Part print with two shaded views. Sizes in mm from the minimum x, y, z corner. A direction names the side the tool comes from. Give positions to 0.01 mm unless a question says otherwise; leave off trailing zeros. Write each loop counter-clockwise with the first axis right and the second up, starting at its lowest first coordinate (ties: lowest second). Pieces come first, ordered by that corner, then holes. Notation, with made-up numbers: M 64,80.25 L 73,80.25 A24 ccw 73,100.25 Z; hole C -39.5,42 d11. An arc over 180 degrees is marked long. Return JSON: item names as keys, results as strings. Group by question number.
Q1. Wall check: probe 1 along X at (y, z) = (1, 3); probe 2 along X at (y, z) = (3.75, 3); probe 3 along Z at (x, y) = (14, 3.5). Give the ranges that are in metal, low to high.
Q2. Band-saw the part on D-D, the plane x = 3.5. Give the cut face in (y, z), then the cut area to 3 significant figures.
Q3. Tool access for the marked faces 4, 5 and 6: list every direction of +Z, -Z, +X, -X, +Y, -Y with a clear straight run to the whole face (end or side of a thin tool).
Q4. Band-saw the part on C-C, the plane z = 3.25. Give the cut face in (x, y).
Q5. Pull direction Z, two halves, no side cores. Call the marked faces 1, 2 and 3: +Z half, -Z half, draft (parallel to the pull), parting line (faces both ways), or undercut.
Q6. Flat gauge pins, fed straight in: pin 1 Ø1.5 at (x, y) = (5.5, 6) entering from -Z; pin 2 Ø5 at (x, y) = (6, 5) entering from +Z; pin 3 Ø1 at (x, y) = (6, 4.5) entering from -Z. Where does each tip first touch, or does it go through?
Q7. Band-saw the part on B-B, the plane y = 4.25. Give the cut face in (x, z).
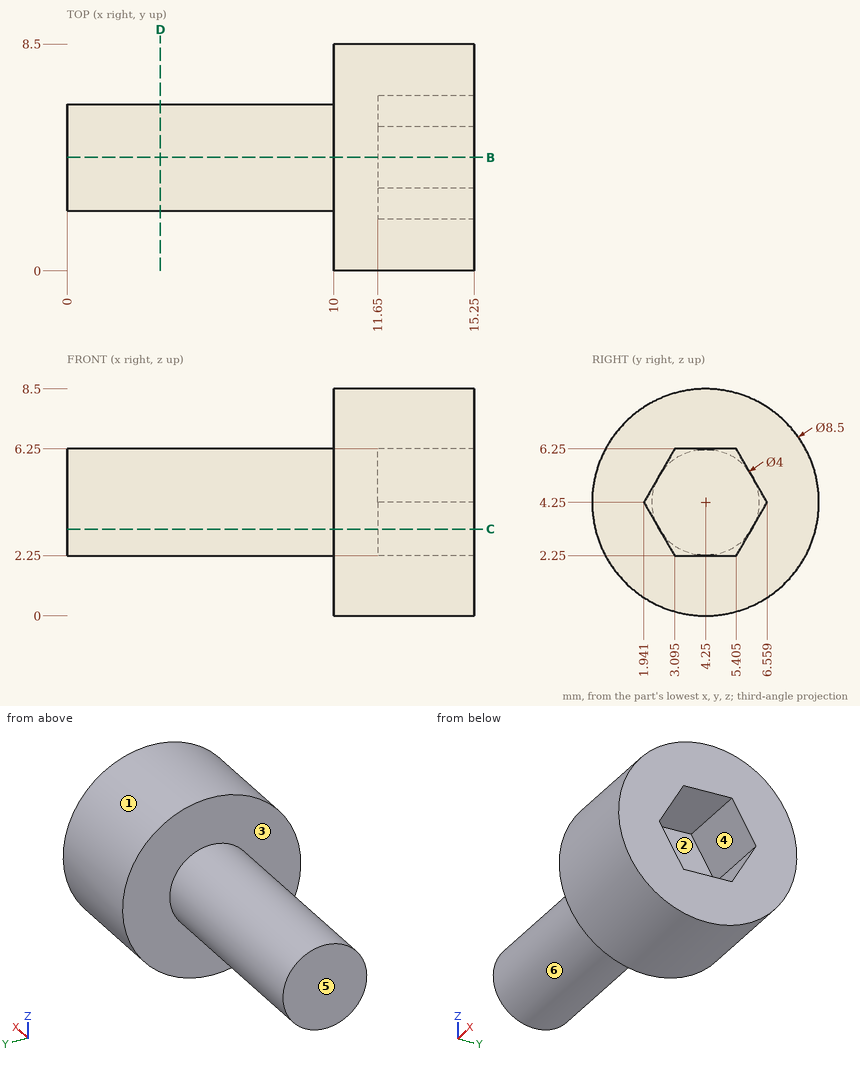
From the geometry:
{
 "1": {"probe 1": "x = 10 to 15.25", "probe 2": "x = 0 to 11.65", "probe 3": "z = 0.07 to 2.25, 6.25 to 8.43"},
 "2": {"outline": "C 4.25,4.25 d4", "area": "12.6 mm^2"},
 "3": {"face 4": "+X", "face 5": "+Z, -Z, -X, +Y, -Y", "face 6": "-X"},
 "4": {"outline": "M 0,2.52 L 10,2.52 L 10,0.12 L 15.25,0.12 L 15.25,2.52 L 11.65,2.52 L 11.65,5.98 L 15.25,5.98 L 15.25,8.38 L 10,8.38 L 10,5.98 L 0,5.98 Z"},
 "5": {"face 1": "parting line", "face 2": "undercut", "face 3": "draft"},
 "6": {"pin 1": "stops at z = 2.52", "pin 2": "stops at z = 6.25", "pin 3": "stops at z = 2.25"},
 "7": {"outline": "M 0,2.25 L 10,2.25 L 10,0 L 15.25,0 L 15.25,2.25 L 11.65,2.25 L 11.65,6.25 L 15.25,6.25 L 15.25,8.5 L 10,8.5 L 10,6.25 L 0,6.25 Z"}
}
